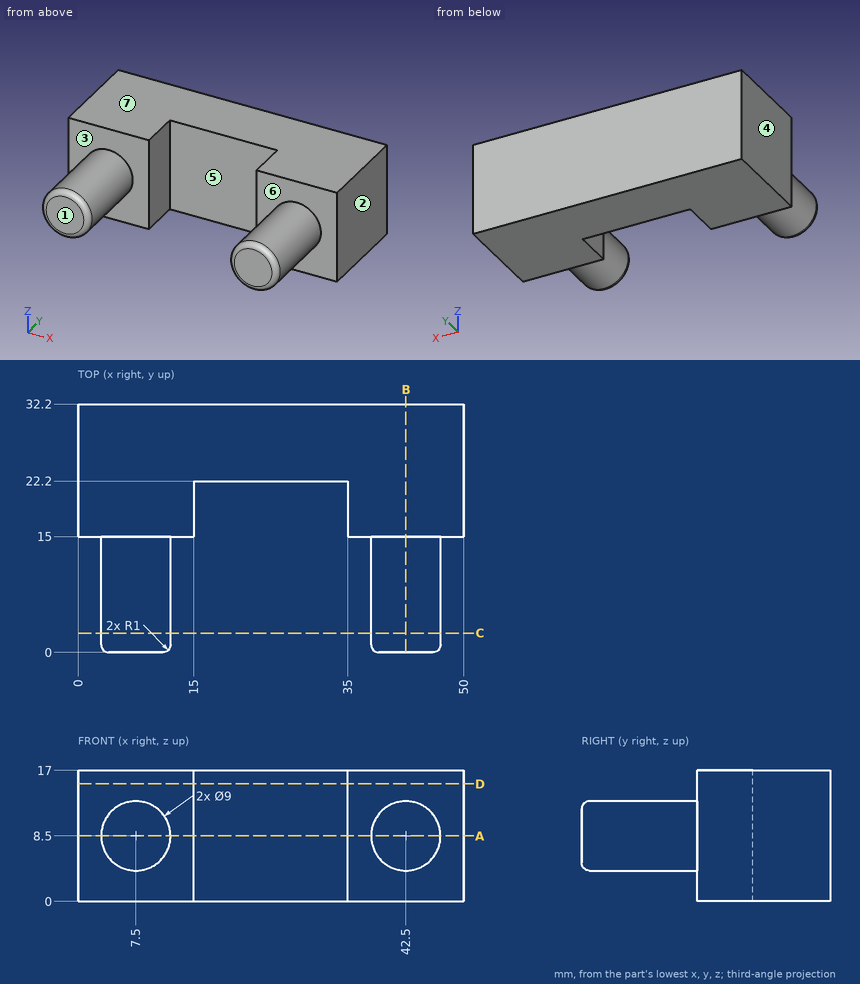
The drawing under review shows one solid part. Ordinate dimensions are in mm from its lowest x, y, z. A direction names the side the tool comes from. Round coordinates to 2 decimals unless told otherwise and drop trailing zeros. Loops run counter-clockwise (first coordinate to the right, second up) from the corner with the lowest first, then second, coordinate; pieces in that order, holes last. Notation, with made-up numbers: (64, -25.5) - (121, -25.5) arc R24 ccw to (121, 11.5) - close; hole circle Ø4 at (36, 37.25). An arc over 180 degrees is marked (long way). One line per item, written item: value. Start each with the question number.
1) Insertion check: pin 1 Ø8 at (y, z) = (18, 7.5) entering from -X; pin 2 Ø10 at (y, z) = (6, 15) entering from -X. Each pin has a flat end and moves straight along its axis. Give the tip position at first contact, or say it passes through.
2) To check wall thickness, follow L1, parallel to X at y = 20.5, z = 15.5; L2, parallel to X at y = 1, z = 8.5; L3, parallel to Y at x = 19, z = 11.75. State the ranges of each line that lie inside material, in increasing order. Write a range as from..to.
3) For the marked faces 5, 6 and 7, list the 3-axis set-ups (+Z, -Z, +X, -X, +Y, -Y) from which the entire face can be reached by the end or side of a thin tool; tool diameter is ignored.
4) Draft analysis for pull direction X (two halves, no side actions). For the marked faces 1, 2, 3 and 4, state which applies: +X half, -X half, draft (parallel to the pull), parting line (faces both ways), or undercut.
5) Consider section C-C on y = 2.5. Give the boundary of the cut face in (x, z), then the cut area to 3 significant figures.
6) Consider section D-D on z = 15.25. Give the boundary of the cut face in (x, y), then the cut area to 3 significant figures.
7) Consider section A-A on z = 8.5. Give the boundary of the cut face in (x, y), then the cut area to 3 significant figures.
8) Consider section B-B on x = 42.5. Give the boundary of the cut face in (y, z), then the cut area to 3 significant figures.
Reported:
1. pin 1: stops at x = 0
1. pin 2: stops at x = 3.26
2. L1: x = 0..15, 35..50
2. L2: x = 3..12, 38..47
2. L3: y = 22.2..32.2
3. face 5: +Z, -Z, -Y
3. face 6: -Y
3. face 7: +Z, +X, -X, +Y, -Y
4. face 1: draft
4. face 2: +X half
4. face 3: undercut
4. face 4: -X half
5. outline: circle Ø9 at (7.5, 8.5); circle Ø9 at (42.5, 8.5)
5. area: 127 mm^2
6. outline: (0, 15) - (15, 15) - (15, 22.2) - (35, 22.2) - (35, 15) - (50, 15) - (50, 32.2) - (0, 32.2) - close
6. area: 716 mm^2
7. outline: (0, 15) - (3, 15) - (3, 1) arc R1 ccw to (4, 0) - (11, 0) arc R1 ccw to (12, 1) - (12, 15) - (15, 15) - (15, 22.2) - (35, 22.2) - (35, 15) - (38, 15) - (38, 1) arc R1 ccw to (39, 0) - (46, 0) arc R1 ccw to (47, 1) - (47, 15) - (50, 15) - (50, 32.2) - (0, 32.2) - close
7. area: 985 mm^2
8. outline: (0, 5) arc R1 ccw to (1, 4) - (15, 4) - (15, 0) - (32.2, 0) - (32.2, 17) - (15, 17) - (15, 13) - (1, 13) arc R1 ccw to (0, 12) - close
8. area: 427 mm^2
